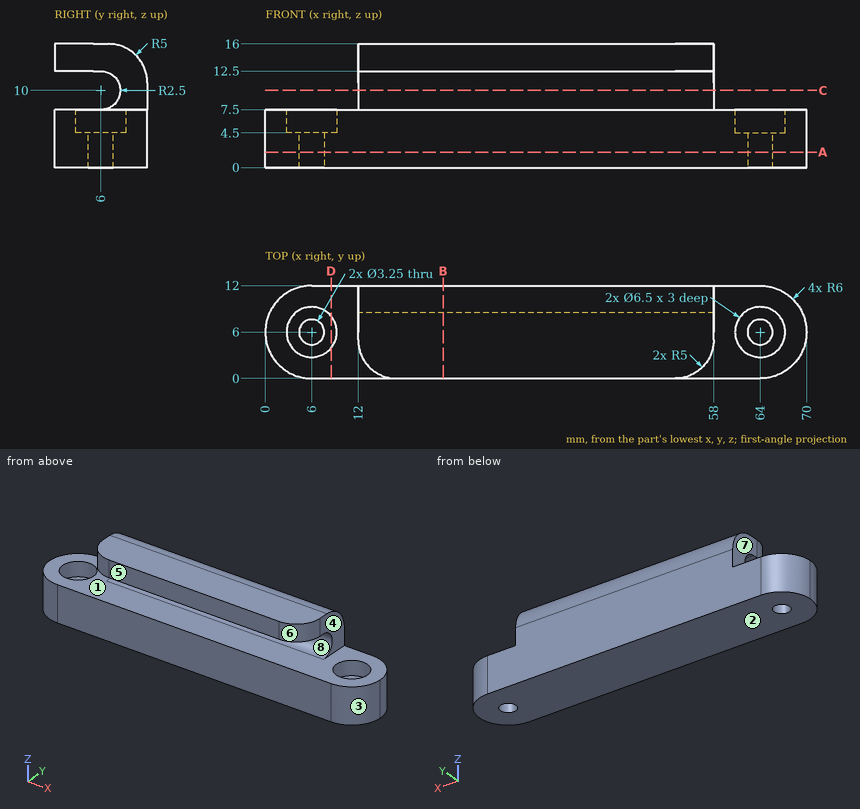
Input: dimensioned drawing with shaded views. Units: mm. Origin: part minimum x, y, z. A direction names the side the tool comes from. Round coordinates to 2 decimals unless told otherwise and drop trailing zeros. Order: outer loops, then holes, each group sorted by start corner. A loop starts at its lowest first (then second) coordinate and runs counter-clockwise, first axis right, second up. Notation, with made-up numbers: (0, -30) -> (26, -30) arc R31 ccw to (26, 4) -> close; hole circle Ø3 at (-8, -23.5). An arc over 180 degrees is marked (long way). Put each result on its own line as item: value. Start each with the question number.
Q1. Section B-B on x = 23. Return the cut outline in (y, z).
Q2. Section C-C on z = 10. Return the cut outline in (x, y).
Q3. Pull-direction query (Z, two-part tool) for the marked faces 1, 2 and 3; classes: +Z half, -Z half, draft (parallel to the pull), parting line (faces both ways), or undercut.
Q4. Line query: probe 1 along Y at (x, z) = (64, 2) (3 decimals); probe 2 along Z at (x, y) = (37, 1); probe 3 along Y at (x, z) = (64, 5.3). Output: solid intervals per line, ascending.
Q5. Section D-D on x = 8.5. Return the cut outline in (y, z), and give its area (3 significant figures).
Q6. Section A-A on z = 2. Give the number of separate pieces and of enclosed holes in the cut face, and give its area (4 significant figures).
Q7. First-contact query: pin 1 (1 mm diameter, centred on y = 9.5, z = 12.5, fed in from +X); pin 2 (1 mm diameter, centred on y = 9, z = 2, fed in from -X); pin 3 (3 mm diameter, centred on x = 33.5, z = 14, fed in from +Y). Flat tips, straight axial feed; report the tip coordinate or a pass-through.
Q8. Reachability of the marked faces 4, 5, 6, 7 and 8 from +Z, -Z, +X, -X, +Y, -Y: full face, straight path, thin tool, end or side. Return the list, or none.
Ans:
1. outline: (0, 0) -> (12, 0) -> (12, 11) arc R5 ccw to (7, 16) -> (0, 16) -> (0, 12.5) -> (6, 12.5) arc R2.5 cw to (6, 7.5) -> (0, 7.5) -> close
2. outline: (12, 8.5) -> (58, 8.5) -> (58, 12) -> (12, 12) -> close
3. face 1: undercut
3. face 2: -Z half
3. face 3: draft
4. probe 1: y = 0 to 4.375, 7.625 to 12
4. probe 2: z = 0 to 7.5, 12.5 to 16
4. probe 3: y = 0 to 2.75, 9.25 to 12
5. outline: (0, 0) -> (12, 0) -> (12, 7.5) -> (8.08, 7.5) -> (8.08, 4.5) -> (3.92, 4.5) -> (3.92, 7.5) -> (0, 7.5) -> close
5. area: 77.5 mm2
6. separate pieces: 1
6. enclosed holes: 2
6. area: 792.5 mm2
7. pin 1: stops at x = 58
7. pin 2: stops at x = 0.55
7. pin 3: stops at y = 11.77
8. face 4: +Z, +X, +Y, -Y
8. face 5: +Z, -Z, +X, -X, -Y
8. face 6: +Z, +X, -Y
8. face 7: +Z, -X, +Y, -Y
8. face 8: +X, -X, -Y
